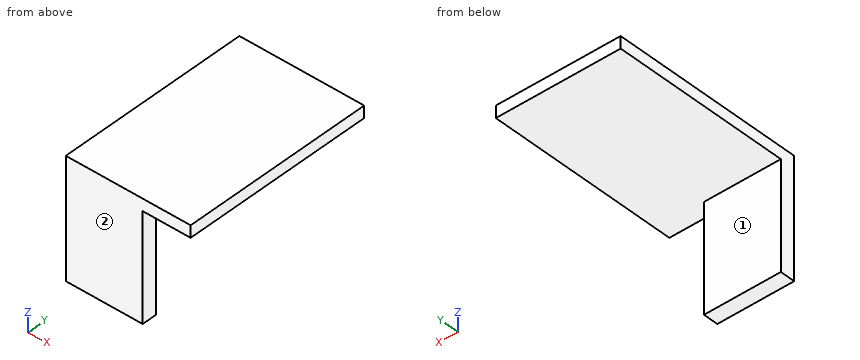
```python
from build123d import *

# Parameters (mm, degrees)
EXTRUDE_1_DEPTH     = 42
SKETCH_3_W          = 16.132543854
SKETCH_3_H          = 36.374490106
CUT_EXTRUDE_1_DEPTH = 82.608823052


with BuildPart() as part:
    # Эскиз1 → Вытянуть1 (new body)
    with BuildSketch(Plane(origin=(0, 0, 0), x_dir=(0, 0, -1), z_dir=(1, 0, 0))):
        Polygon((0, 0), (0, 60), (-4, 60), (-4, -5), (36, -5), (36, 0), align=None)
    extrude(amount=-EXTRUDE_1_DEPTH)

    # Эскиз3 → Вырез-Вытянуть1 (cut, through all)
    with BuildSketch(Plane(origin=(0, 0, 0), x_dir=(1, 0, 0), z_dir=(0, 1, 0))):
        with Locations((-8.066271927, 18.187245053)):
            Rectangle(SKETCH_3_W, SKETCH_3_H)
    extrude(amount=-CUT_EXTRUDE_1_DEPTH, mode=Mode.SUBTRACT)


solid = part.part
```
Design review of the part built by this model. Coordinates are the model's own, in mm. Face numbers are marked on the shaded views. A direction names the side the tool comes from. Coordinates: 2 decimals unless noted, no trailing zeros. Write each loop counter-clockwise with the first axis right and the second up, starting at its lowest first coordinate (ties: lowest second). Pieces come first, ordered by that corner, then holes.
1) Add section C-C (y = 9). Write out the cut boundary in (x, z), plus the area to 3 significant figures.
2) To check wall thickness, follow L1, parallel to Z at x = -24, y = 6.5; L2, parallel to Y at x = -18.5, z = -31. State the ranges of each line that lie inside material, in increasing order.
3) Add section A-A (x = -36). Write out the cut boundary in (y, z), plus the area to 3 significant figures.
4) Add section B-B (z = -15.5). Write out the cut boundary in (x, y), plus the area to 3 significant figures.
5) Insertion check: pin 1 (12.5 mm diameter, centred on x = -31, y = 23.5, fed in from -Z); pin 2 (2 mm diameter, centred on x = -18, z = -26.5, fed in from +Y); pin 3 (5.5 mm diameter, centred on y = -2.5, z = -25.5, fed in from +X). Each pin has a flat end and moves straight along its axis. Give the tip position at first contact, or say it passes through.
6) Machinability: for the marked faces 1 and 2, which of the approach directions +Z, -Z, +X, -X, +Y, -Y give a long, thin tool a straight path to every point of the face, cutting with its end or side? Answer none if there is none.
Check result:
1. outline: (-42, 0) - (0, 0) - (0, 4) - (-42, 4) - close
1. area: 168 mm2
2. L1: z = 0 to 4
2. L2: y = -5 to 0
3. outline: (-5, -36) - (0, -36) - (0, 0) - (60, 0) - (60, 4) - (-5, 4) - close
3. area: 440 mm2
4. outline: (-42, -5) - (-16.13, -5) - (-16.13, 0) - (-42, 0) - close
4. area: 129 mm2
5. pin 1: stops at z = 0
5. pin 2: stops at y = 0
5. pin 3: stops at x = -16.13
6. face 1: -Z, +X, -X, +Y
6. face 2: +Z, -Z, +X, -X, -Y
